Verification items for this drawing (mm, ordinates from the low corner). A direction names the side the tool comes from. Give positions to 0.01 mm unless a question says otherwise; leave off trailing zeros. Write each loop counter-clockwise with the first axis right and the second up, starting at its lowest first coordinate (ties: lowest second). Pieces come first, ordered by that corner, then holes. Notation, with made-up numbers: (-0.5, -40) -> (21.5, -40) arc R34 cw to (21.5, -6) -> close; hole circle Ø8 at (85, 59). An arc over 180 degrees is marked (long way). Answer as a JSON object with one key per item and string values.
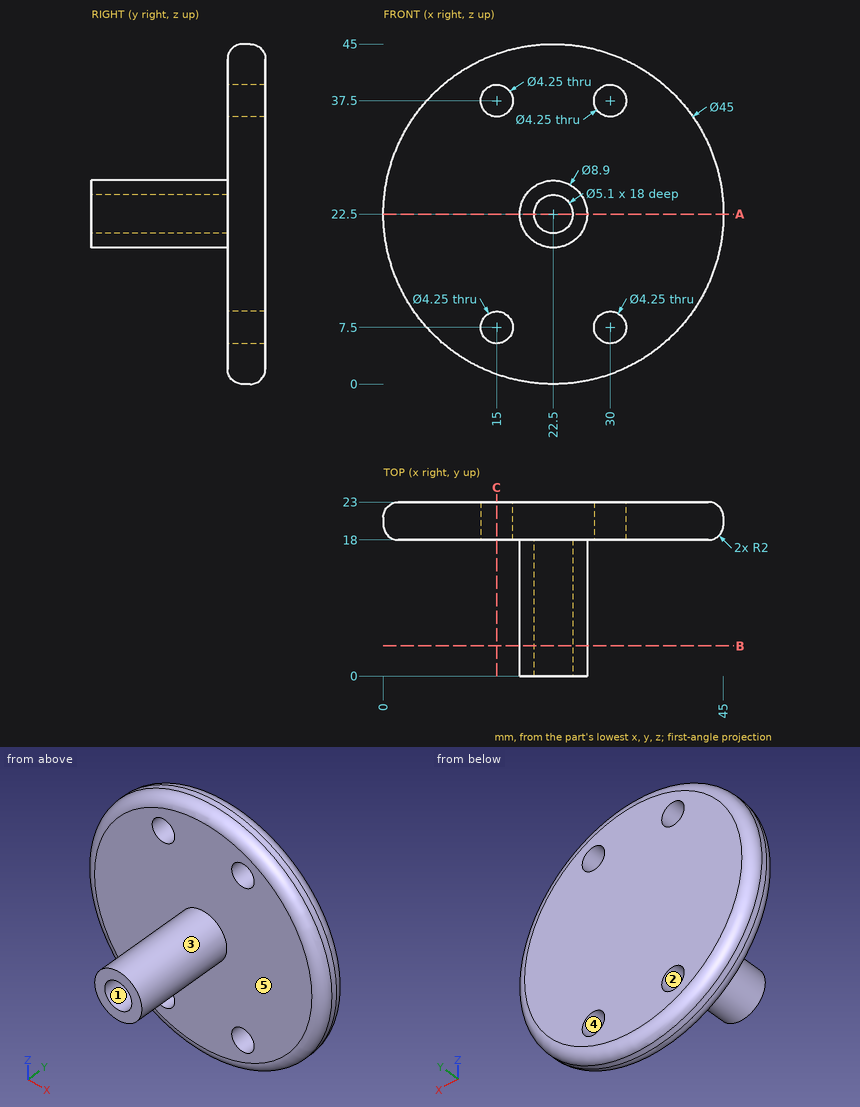
1. Access from +Z, -Z, +X, -X, +Y, -Y to the whole of each face (thin tool, end or side, straight path). Record for the marked faces 1 and 2.
Determined:
{"face 1": "-Y", "face 2": "+Y, -Y"}
2. Go/stop test with a flat-tipped pin: P1, Ø6, axis at x = 24.5, z = 32, coming from the -Y side. Record where the tip stops, or that it passes through.
Determined:
{"P1": "y = 18"}
3. Sectioned sample at C-C, the plane x = 15. State how many separate pieces and enclosed holes the cut face has, plus the area to 3 significant figures.
Determined:
{"separate pieces": "3", "enclosed holes": "0", "area": "166 mm^2"}
4. Sectioned sample at A-A, the plane z = 22.5. Enter the section's corners in (x, y), plus the area to 3 significant figures.
Determined:
{"outline": "(0, 20) arc R2 ccw to (2, 18) -> (18.05, 18) -> (18.05, 0) -> (19.95, 0) -> (19.95, 18) -> (25.05, 18) -> (25.05, 0) -> (26.95, 0) -> (26.95, 18) -> (43, 18) arc R2 ccw to (45, 20) -> (45, 21) arc R2 ccw to (43, 23) -> (2, 23) arc R2 ccw to (0, 21) -> close", "area": "290 mm^2"}
5. Sectioned sample at B-B, the plane y = 4. Enter the section's corners in (x, z), plus the area to 3 significant figures.
Determined:
{"outline": "circle Ø8.9 at (22.5, 22.5); hole circle Ø5.1 at (22.5, 22.5)", "area": "41.8 mm^2"}
6. Mould release check, pull along X, two halves, no side actions. Record for the marked faces 3, 4 and 5: released by +X, released by -X, zero draft, split by the parting line, or undercut.
Determined:
{"face 3": "split by the parting line", "face 4": "undercut", "face 5": "zero draft"}
7. Scan lines: L1, parallel to X at y = 19.75, z = 38; L2, parallel to Z at x = 15, y = 19.8 (3 decimals); L3, parallel to Z at x = 29, y = 20.5 (3 decimals). Record each from-to range of solid material in increasing order. Write a range as [from, to].
Determined:
{"L1": "[6.21, 12.93], [17.07, 27.93], [32.07, 38.79]", "L2": "[1.297, 5.375], [9.625, 35.375], [39.625, 43.703]", "L3": "[0.959, 5.625], [9.375, 35.625], [39.375, 44.041]"}
